Source: CAD feature listing. Evaluate the final solid. Frame: model axes, mm. A direction names the side the tool comes from. Coordinates: 2 decimals unless noted, no trailing zeros. Write each loop counter-clockwise with the first axis right and the second up, starting at its lowest first coordinate (ties: lowest second). Pieces come first, ordered by that corner, then holes. Notation, with made-up numbers: M 79,-19.75 L 120,-19.75 A37 ccw 120,16.25 Z; hole C 5.25,-14.5 d2. An arc over 180 degrees is marked long. One line per item, written item: value. Start each with the question number.
Item 1: Cut plane C-C, the plane z = 20.5. Output: boundary loops of the cut face in (x, y), then the cut area to 3 significant figures.
Item 2: Set-up query: faces 1 (the flat face through (0, 0, 0)), 2 (the cylindrical face through (1.172, 8.923, 0.986)). Return all of +Z, -Z, +X, -X, +Y, -Y with unobstructed straight access to the full face (end or side cutting, diameter ignored); none if empty.
Item 3: Cut plane A-A, the plane x = 0. Output: boundary loops of the cut face in (y, z), then the cut area to 3 significant figures.
Item 4: Pin query (flat end, axial travel): P1, Ø7, axis at x = 4, y = 0.5, coming from the -Z side; P2, Ø1.5, axis at x = 3.5, z = 7, coming from the +Y side; P3, Ø8, axis at x = -7.5, z = 10.5, coming from the +Y side; P4, Ø1, axis at y = 8, z = 8.5, coming from the +X side. Return the tip coordinate at first contact, or that it passes through.
Item 5: Ray query, L1, parallel to Y at x = 0, z = 0.95; L2, parallel to X at y = -0.25, z = 18.25; L3, parallel to Z at x = 5.5, y = 6.75. Return the intervals inside material, ascending. Write a range as from..to.
Item 6: Mould query, pull axis Y, two halves, no side actions, for faces 3 (the cylindrical face through (-1.269, 9.667, 11.832)), 4 (the cylindrical face through (1.73, -7.81, 0.99)), 5 (the flat face through (-9, 5, 24)). Classes: released by +Y, released by -Y, zero draft, split by the parting line, or undercut.
```python
from build123d import *

# Parameters (mm, degrees)
SKETCH1_R           = 9.75
BOSS_EXTRUDE1_DEPTH = 24
SKETCH3_R           = 11.5
BOSS_EXTRUDE2_DEPTH = 2
SKETCH4_R           = 9
SKETCH4_R_2         = 8
CUT_EXTRUDE1_DEPTH  = 2


with BuildPart() as part:
    # Sketch1 → Boss-Extrude1 (new body)
    with BuildSketch(Plane.XY):
        Circle(SKETCH1_R)
    extrude(amount=BOSS_EXTRUDE1_DEPTH)

    # Sketch3 → Boss-Extrude2 (add)
    with BuildSketch(Plane.XY.offset(24)):
        Circle(SKETCH3_R)
    extrude(amount=BOSS_EXTRUDE2_DEPTH)

    # Sketch4 → Cut-Extrude1 (cut)
    with BuildSketch(Plane(origin=(0, 0, 0), x_dir=(-1, 0, 0), z_dir=(0, 0, -1))):
        Circle(SKETCH4_R)
        Circle(SKETCH4_R_2, mode=Mode.SUBTRACT)
    extrude(amount=-CUT_EXTRUDE1_DEPTH, mode=Mode.SUBTRACT)


solid = part.part
```
From the geometry:
1. outline: C 0,0 d19.5
1. area: 299 mm²
2. face 1: -Z, +X, -X, +Y, -Y
2. face 2: -Z
3. outline: M -11.5,24 L -9.75,24 L -9.75,0 L -9,0 L -9,2 L -8,2 L -8,0 L 8,0 L 8,2 L 9,2 L 9,0 L 9.75,0 L 9.75,24 L 11.5,24 L 11.5,26 L -11.5,26 Z
3. area: 510 mm²
4. P1: stops at z = 0
4. P2: stops at y = 9.35
4. P3: stops at y = 9.1
4. P4: stops at x = 6.23
5. L1: y = -9.75..-9, -8..8, 9..9.75
5. L2: x = -9.75..9.75
5. L3: z = 2..26
6. face 3: split by the parting line
6. face 4: undercut
6. face 5: zero draft
